The figure shows three views and two pictorial views of one solid part (mm, origin at its lowest corner). Answer the questions. A direction names the side the tool comes from. Round coordinates to 2 decimals unless told otherwise and drop trailing zeros. Write each loop counter-clockwise with the first axis right and the second up, starting at its lowest first coordinate (ties: lowest second). Pieces come first, ordered by that corner, then holes. Notation, with made-up numbers: (43.5, 86) -> (52.5, 86) arc R28 cw to (52.5, 111) -> close; hole circle Ø10 at (81, 34). An arc over 180 degrees is marked (long way). One line per item, written item: value.
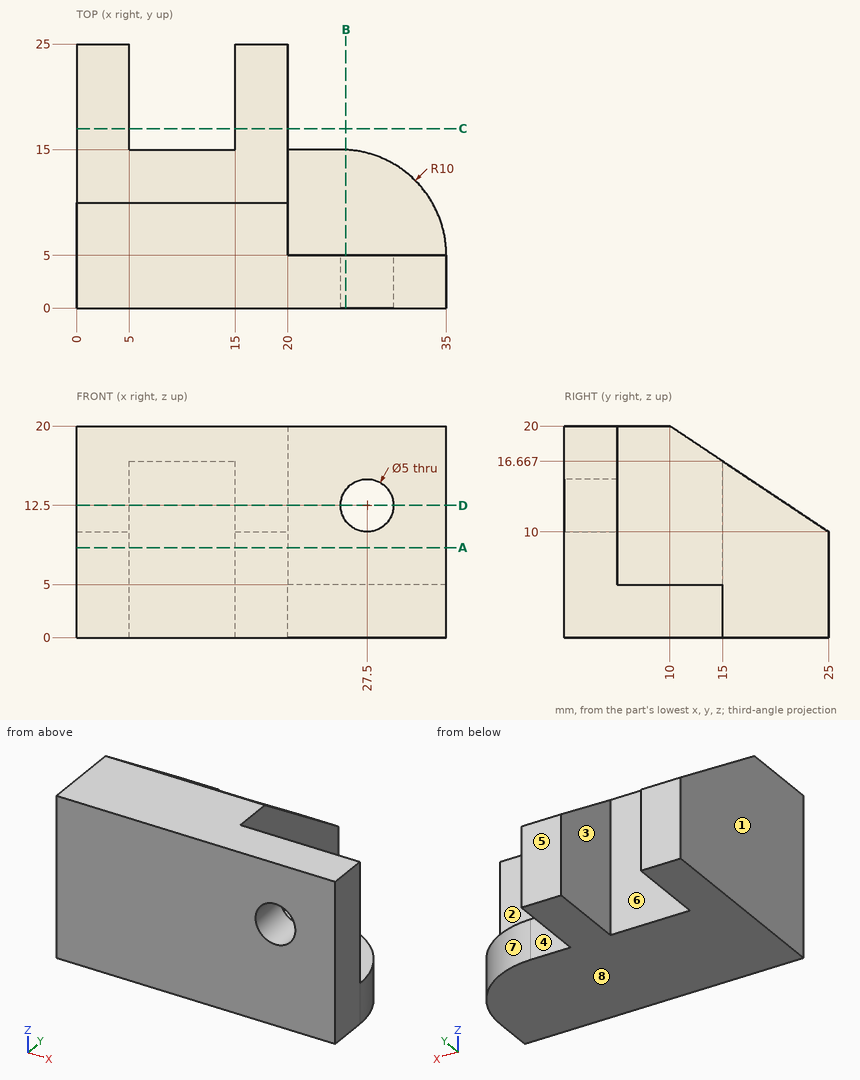
(1) Find section C-C on y = 17. Give the vertices of the cut face in (x, z).
Reported:
outline: (0, 0) -> (5, 0) -> (5, 15.33) -> (0, 15.33) -> close; (15, 0) -> (20, 0) -> (20, 15.33) -> (15, 15.33) -> close
(2) Flat-ended cylindrical pins translate along their axes: pin 1 Ø3 at (x, z) = (21.5, 2) entering from -Y; pin 2 Ø7.5 at (x, z) = (31, 16) entering from +Y; pin 3 Ø5 at (x, z) = (9.5, 6) entering from +Y; pin 4 Ø5 at (x, y) = (26.5, 9.5) entering from +Z. Find the tip coordinate at first contact, or state that the pin passes through.
Reported:
pin 1: stops at y = 0
pin 2: stops at y = 5
pin 3: stops at y = 15
pin 4: stops at z = 5
(3) A tool of negligible diameter and unlimited length cuts with its end or side. For the marked faces 1, 2, 3, 4 and 5, from which of +Z, -Z, +X, -X, +Y, -Y can it reach the whole face along a straight path? Write none if from no direction.
Reported:
face 1: +Z, -Z, -X, +Y, -Y
face 2: +Z, +X, +Y
face 3: +Z, -Z, +Y
face 4: +Z, -Z, +X, +Y
face 5: +Z, -Z, +X, -X, +Y
(4) Find section A-A on z = 8.5. Give the vertices of the cut face in (x, y).
Reported:
outline: (0, 0) -> (35, 0) -> (35, 5) -> (20, 5) -> (20, 25) -> (15, 25) -> (15, 15) -> (5, 15) -> (5, 25) -> (0, 25) -> close
(5) Consider probe 1 along X at (y, z) = (3.85, 12.5); probe 2 along X at (y, z) = (19.5, 10); probe 3 along Y at (x, z) = (32, 7.5). Determine where each line is inside the solid, lowest interval first.
Reported:
probe 1: x = 0 to 25, 30 to 35
probe 2: x = 0 to 5, 15 to 20
probe 3: y = 0 to 5
(6) For a pull along X with two mould halves and no side action, classify the marked faces 6, 7 and 8 as pulls with the +X half, pulls with the -X half, needs draft (parallel to the pull), parting line crosses it, or undercut.
Reported:
face 6: undercut
face 7: pulls with the +X half
face 8: needs draft
(7) Find section B-B on x = 25.5. Give the vertices of the cut face in (y, z).
Reported:
outline: (0, 0) -> (14.99, 0) -> (14.99, 5) -> (5, 5) -> (5, 11) -> (0, 11) -> close; (0, 14) -> (5, 14) -> (5, 20) -> (0, 20) -> close
(8) Find section D-D on z = 12.5. Give the vertices of the cut face in (x, y).
Reported:
outline: (0, 0) -> (25, 0) -> (25, 5) -> (20, 5) -> (20, 21.25) -> (15, 21.25) -> (15, 15) -> (5, 15) -> (5, 21.25) -> (0, 21.25) -> close; (30, 0) -> (35, 0) -> (35, 5) -> (30, 5) -> close
